The model under review builds one solid part; all positions refer to its coordinate system, in mm. Coordinates: 2 decimals unless noted, no trailing zeros. Write each loop counter-clockwise with the first axis right and the second up, starting at its lowest first coordinate (ties: lowest second). Pieces come first, ordered by that corner, then holes.
```python
from build123d import *

# Parameters (mm, degrees)
SKETCH1_R                = 54.5
BOSS_EXTRUDE1_DEPTH      = 1.5
SKETCH2_R                = 1
CUT_EXTRUDE1_DEPTH       = 1.58
SKICA1_W                 = 7.7
SKICA1_H                 = 32
ODEBRAT_VYSUNUT_M1_DEPTH = 1.5


with BuildPart() as part:
    # Sketch1 → Boss-Extrude1 (new body)
    with BuildSketch(Plane.XY):
        Circle(SKETCH1_R)
    extrude(amount=BOSS_EXTRUDE1_DEPTH)

    # Sketch2 → Cut-Extrude1 (cut)
    with BuildSketch(Plane.XY.offset(1.5)):
        with Locations((29.900398584, 26.1)):
            Circle(SKETCH2_R)
        with Locations((29.900398584, -33.3)):
            Circle(SKETCH2_R)
        with Locations((-29.999601416, -33.3)):
            Circle(SKETCH2_R)
        with Locations((-29.999601416, 26.1)):
            Circle(SKETCH2_R)
    extrude(amount=-CUT_EXTRUDE1_DEPTH, mode=Mode.SUBTRACT)

    # Skica1 → Odebrat vysunutím1 (cut)
    with BuildSketch(Plane.XY.offset(1.5)):
        with Locations((41.7205, 0)):
            Rectangle(SKICA1_W, SKICA1_H)
        with Locations((-41.7205, 0)):
            Rectangle(SKICA1_W, SKICA1_H)
    extrude(amount=-ODEBRAT_VYSUNUT_M1_DEPTH, mode=Mode.SUBTRACT)


solid = part.part
```
Item 1: To check wall thickness, follow line 1 along Y through (x, z) = (39, 0.95); line 2 along Y through (x, z) = (-42, 0.45); line 3 along X through (y, z) = (12.5, 0.7). State the ranges of each line that lie inside material, in increasing order.
Solved:
line 1: y = -38.07 to -16, 16 to 38.07
line 2: y = -34.73 to -16, 16 to 34.73
line 3: x = -53.05 to -45.57, -37.87 to 37.87, 45.57 to 53.05
Item 2: Take a section at D-D, the plane x = 16. Write out the cut boundary in (y, z).
Solved:
outline: (-52.1, 0) - (52.1, 0) - (52.1, 1.5) - (-52.1, 1.5) - close
Item 3: Take a section at A-A, the plane y = 13.5. Write out the cut boundary in (x, z).
Solved:
outline: (-52.8, 0) - (-45.57, 0) - (-45.57, 1.5) - (-52.8, 1.5) - close; (-37.87, 0) - (37.87, 0) - (37.87, 1.5) - (-37.87, 1.5) - close; (45.57, 0) - (52.8, 0) - (52.8, 1.5) - (45.57, 1.5) - close
Item 4: Take a section at B-B, the plane z = 0.45. Write out the cut boundary in (x, y), plus the area to 3 significant figures.
Solved:
outline: circle Ø109 at (0, 0); hole (-45.57, -16) - (-37.87, -16) - (-37.87, 16) - (-45.57, 16) - close; hole circle Ø2 at (-30, -33.3); hole circle Ø2 at (-30, 26.1); hole circle Ø2 at (29.9, -33.3); hole circle Ø2 at (29.9, 26.1); hole (37.87, -16) - (45.57, -16) - (45.57, 16) - (37.87, 16) - close
area: 8,830 mm2
Item 5: Take a section at C-C, the plane x = -34.5. Write out the cut boundary in (y, z), plus the area to 3 significant figures.
Solved:
outline: (-42.19, 0) - (42.19, 0) - (42.19, 1.5) - (-42.19, 1.5) - close
area: 127 mm2
Item 6: For pin 1 (0.8 mm diameter, centred on y = -3, z = 0.5, fed in from +X); pin 2 (0.8 mm diameter, centred on x = 43.5, z = 1, fed in from +Y); pin 3 (0.8 mm diameter, centred on x = -40.5, z = 0.5, fed in from -Y), all flat-tipped, find the tip position at first contact; note any pin that passes through.
Solved:
pin 1: stops at x = 54.44
pin 2: stops at y = 33.36
pin 3: stops at y = -36.91
